Design review of the part built by this model. Coordinates are the model's own, in mm. Face numbers are marked on the shaded views. A direction names the side the tool comes from. Coordinates: 2 decimals unless noted, no trailing zeros. Loops run counter-clockwise (first coordinate to the right, second up) from the corner with the lowest first, then second, coordinate; pieces in that order, holes last. Notation, with made-up numbers: (32.5, 16) -> (46.5, 16) arc R16 ccw to (46.5, 34) -> close; hole circle Ø10 at (48.25, 74). An arc over 180 degrees is marked (long way). One line per item, written item: value. Start each with the question number.
1. Add section B-B on y = -8. Write out the cut boundary in (x, z) (3 decimals).
2. Machinability: for the marked faces 1 and 2, which of the approach directions +Z, -Z, +X, -X, +Y, -Y give a long, thin tool a straight path to every point of the face, cutting with its end or side? Answer none if there is none.
3. Add section A-A on z = 53. Write out the cut boundary in (x, y) (3 decimals), plus the area to 3 significant figures.
4. Add section D-D on y = 0. Write out the cut boundary in (x, z) (3 decimals).
5. Insertion check: pin 1 (11.5 mm diameter, centred on y = -8, z = 27, fed in from +X); pin 2 (3 mm diameter, centred on x = -21.5, y = 1.5, fed in from +Z) (3 decimals); pin 3 (8 mm diameter, centred on x = 20.5, z = 9, fed in from -Y). Each pin has a flat end and moves straight along its axis. Give the tip position at first contact, or say it passes through.
6. Add section C-C on x = -14. Write out the cut boundary in (y, z) (3 decimals).
7. For probe 1 along Y at (x, z) = (-16, 1.5) (3 decimals); probe 2 along X at (y, z) = (12, 16); probe 3 along Z at (x, y) = (-10, -14.5) (3 decimals), list the stretches that pass through material, from the lowest coordinate up.
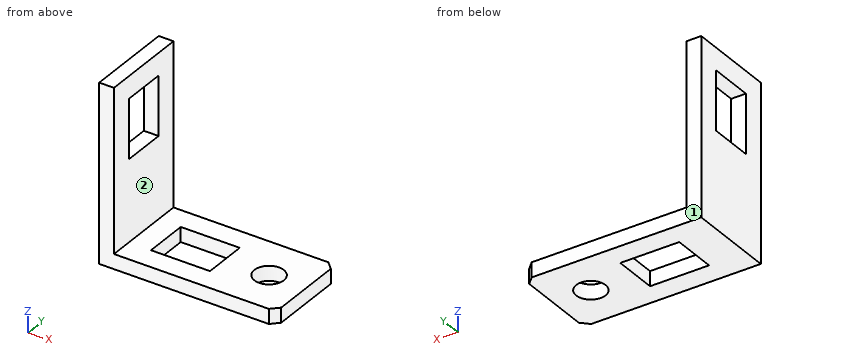
```python
from build123d import *

# Parameters (mm, degrees)
SKETCH1_W           = 6.35
SKETCH1_H           = 69.85
SKETCH1_W_2         = 76.2
SKETCH1_H_2         = 6.35
BOSS_EXTRUDE1_DEPTH = 19.05
SKETCH2_R           = 6.35
CUT_EXTRUDE1_DEPTH  = 6.35
SKETCH3_W           = 25.4
SKETCH3_H           = 19.05
CUT_EXTRUDE2_DEPTH  = 6.35
CUT_EXTRUDE3_DEPTH  = 6.35
SKETCH5_W           = 25.4
SKETCH5_H           = 19.05
CUT_EXTRUDE4_DEPTH  = 6.35


with BuildPart() as part:
    # Sketch1 → Boss-Extrude1 (new, symmetric)
    with BuildSketch(Plane(origin=(0, 0, 0), x_dir=(1, 0, 0), z_dir=(0, 1, 0))):
        with Locations((-34.925, -38.1)):
            Rectangle(SKETCH1_W, SKETCH1_H)
        Rectangle(SKETCH1_W_2, SKETCH1_H_2)
    extrude(amount=BOSS_EXTRUDE1_DEPTH, both=True)

    # Sketch2 → Cut-Extrude1 (cut)
    with BuildSketch(Plane(origin=(0, 0, -3.175), x_dir=(-1, 0, 0), z_dir=(0, 0, -1))):
        with Locations((-22.225, 0)):
            Circle(SKETCH2_R)
    extrude(amount=-CUT_EXTRUDE1_DEPTH, mode=Mode.SUBTRACT)

    # Sketch3 → Cut-Extrude2 (cut)
    with BuildSketch(Plane(origin=(0, 0, -3.175), x_dir=(-1, 0, 0), z_dir=(0, 0, -1))):
        with Locations((9.525, 0)):
            Rectangle(SKETCH3_W, SKETCH3_H)
    extrude(amount=-CUT_EXTRUDE2_DEPTH, mode=Mode.SUBTRACT)

    # Sketch4 → Cut-Extrude3 (cut)
    with BuildSketch(Plane(origin=(0, 0, -3.175), x_dir=(-1, 0, 0), z_dir=(0, 0, -1))):
        Polygon((-34.925, 19.05), (-38.1, 15.875), (-38.1, 19.05), align=None)
        Polygon((-34.925, -19.05), (-38.1, -15.875), (-38.1, -19.05), align=None)
    extrude(amount=-CUT_EXTRUDE3_DEPTH, mode=Mode.SUBTRACT)

    # Sketch5 → Cut-Extrude4 (cut)
    with BuildSketch(Plane(origin=(-31.75, 0, 0), x_dir=(0, 0, -1), z_dir=(1, 0, 0))):
        with Locations((-50.8, 0)):
            Rectangle(SKETCH5_W, SKETCH5_H)
    extrude(amount=-CUT_EXTRUDE4_DEPTH, mode=Mode.SUBTRACT)


solid = part.part
```
Worked answers:
1. outline: (-38.1, -3.175) -> (-22.225, -3.175) -> (-22.225, 3.175) -> (-31.75, 3.175) -> (-31.75, 38.1) -> (-38.1, 38.1) -> close; (-38.1, 63.5) -> (-31.75, 63.5) -> (-31.75, 73.025) -> (-38.1, 73.025) -> close; (3.175, -3.175) -> (38.1, -3.175) -> (38.1, 3.175) -> (3.175, 3.175) -> close
2. face 1: +Z, -Z, +X, -X, +Y
2. face 2: +Z, +X, +Y, -Y
3. outline: (-38.1, -19.05) -> (-31.75, -19.05) -> (-31.75, -9.525) -> (-38.1, -9.525) -> close; (-38.1, 9.525) -> (-31.75, 9.525) -> (-31.75, 19.05) -> (-38.1, 19.05) -> close
3. area: 121 mm²
4. outline: (-38.1, -3.175) -> (-22.225, -3.175) -> (-22.225, 3.175) -> (-31.75, 3.175) -> (-31.75, 38.1) -> (-38.1, 38.1) -> close; (-38.1, 63.5) -> (-31.75, 63.5) -> (-31.75, 73.025) -> (-38.1, 73.025) -> close; (3.175, -3.175) -> (15.875, -3.175) -> (15.875, 3.175) -> (3.175, 3.175) -> close; (28.575, -3.175) -> (38.1, -3.175) -> (38.1, 3.175) -> (28.575, 3.175) -> close
5. pin 1: stops at x = -31.75
5. pin 2: stops at z = 3.175
5. pin 3: passes through
6. outline: (-19.05, -3.175) -> (-9.525, -3.175) -> (-9.525, 3.175) -> (-19.05, 3.175) -> close; (9.525, -3.175) -> (19.05, -3.175) -> (19.05, 3.175) -> (9.525, 3.175) -> close
7. probe 1: y = -19.05 to -9.525, 9.525 to 19.05
7. probe 2: x = -38.1 to -31.75
7. probe 3: z = -3.175 to 3.175
